Model file for the job. Use its own axes, mm. Face numbers are marked on the shaded views. Give positions to 0.01 mm unless a question says otherwise; leave off trailing zeros. Write each loop counter-clockwise with the first axis right and the second up, starting at its lowest first coordinate (ties: lowest second). Pieces come first, ordered by that corner, then holes. Notation, with made-up numbers: (23.25, 71.25) - (29.25, 71.25) arc R15 cw to (29.25, 80.25) - close; hole circle Ø6 at (11.5, 46). An arc over 180 degrees is marked (long way). Use CSV: the item, a comma, the result in double quotes.
from build123d import *

# Parameters (mm, degrees)
SKETCH1_W               = 245
SKETCH1_H               = 245
BOSS_EXTRUDE1_DEPTH     = 5
SKETCH2_R               = 16.25
CUT_EXTRUDE1_DEPTH      = 10
SKETCH3_R               = 9
CUT_EXTRUDE2_DEPTH      = 10
SKETCH3_3_R             = 9
CUT_EXTRUDE3_DEPTH      = 6
CUT_EXTRUDE3_DEPTH_BACK = 6


with BuildPart() as part:
    # Sketch1 → Boss-Extrude1 (new body, symmetric)
    with BuildSketch(Plane(origin=(0, 0, 0), x_dir=(1, 0, 0), z_dir=(0, 1, 0))):
        Rectangle(SKETCH1_W, SKETCH1_H)
    extrude(amount=BOSS_EXTRUDE1_DEPTH, both=True)

    # Sketch2 → Cut-Extrude1 (cut)
    with BuildSketch(Plane(origin=(0, 5, 0), x_dir=(1, 0, 0), z_dir=(0, 1, 0))):
        with Locations((-66.25, 76.25)):
            Circle(SKETCH2_R)
        with Locations((66.25, 76.25)):
            Circle(SKETCH2_R)
    extrude(amount=-CUT_EXTRUDE1_DEPTH, mode=Mode.SUBTRACT)

    # Sketch3 → Cut-Extrude2 (cut)
    with BuildSketch(Plane(origin=(0, 0, 0), x_dir=(1, 0, 0), z_dir=(0, 1, 0))):
        with Locations((71.5, -103.5)):
            Circle(SKETCH3_R)
    extrude(amount=-CUT_EXTRUDE2_DEPTH, mode=Mode.SUBTRACT)

    # Sketch3<3> → Cut-Extrude3 (cut, two sides)
    with BuildSketch(Plane(origin=(0, 0, 0), x_dir=(1, 0, 0), z_dir=(0, 1, 0))) as cut_extrude3_sk:
        with Locations((103.5, -88.5)):
            Circle(SKETCH3_3_R)
        with Locations((71.5, -103.5)):
            Circle(SKETCH3_3_R)
        with Locations((-71.5, -103.5)):
            Circle(SKETCH3_3_R)
        with Locations((-103.5, -88.5)):
            Circle(SKETCH3_3_R)
    extrude(amount=CUT_EXTRUDE3_DEPTH, mode=Mode.SUBTRACT)
    extrude(cut_extrude3_sk.sketch, amount=-CUT_EXTRUDE3_DEPTH_BACK, mode=Mode.SUBTRACT)


solid = part.part
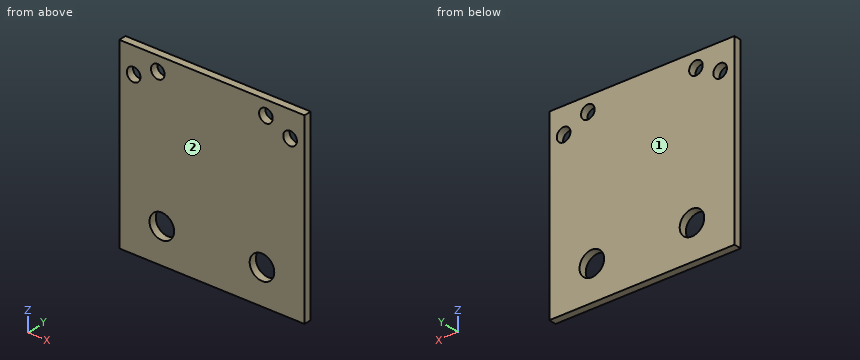
(1) Saw through at A-A, the plane z = 88.5. List the corners of the cut face in (x, y), then the cut area to 3 significant figures.
Checked values:
outline,"(-122.5, -5) - (-112.5, -5) - (-112.5, 5) - (-122.5, 5) - close; (-94.5, -5) - (94.5, -5) - (94.5, 5) - (-94.5, 5) - close; (112.5, -5) - (122.5, -5) - (122.5, 5) - (112.5, 5) - close"
area,"2,090 mm^2"
(2) Saw through at D-D, the plane z = -76.25. List the corners of the cut face in (x, y), then the cut area to 3 significant figures.
Checked values:
outline,"(-122.5, -5) - (-82.5, -5) - (-82.5, 5) - (-122.5, 5) - close; (-50, -5) - (50, -5) - (50, 5) - (-50, 5) - close; (82.5, -5) - (122.5, -5) - (122.5, 5) - (82.5, 5) - close"
area,"1,800 mm^2"
(3) Saw through at C-C, the plane x = -103.5. List the corners of the cut face in (y, z), then the cut area to 3 significant figures.
Checked values:
outline,"(-5, -122.5) - (5, -122.5) - (5, 79.5) - (-5, 79.5) - close; (-5, 97.5) - (5, 97.5) - (5, 122.5) - (-5, 122.5) - close"
area,"2,270 mm^2"
(4) Saw through at B-B, the plane y = 3. List the corners of the cut face in (x, z), then the cut area to 3 significant figures.
Checked values:
outline,"(-122.5, -122.5) - (122.5, -122.5) - (122.5, 122.5) - (-122.5, 122.5) - close; hole circle Ø18 at (-103.5, 88.5); hole circle Ø32.5 at (-66.25, -76.25); hole circle Ø18 at (-71.5, 103.5); hole circle Ø32.5 at (66.25, -76.25); hole circle Ø18 at (71.5, 103.5); hole circle Ø18 at (103.5, 88.5)"
area,"57,300 mm^2"
(5) Pull direction Y, two halves, no side cores. Call the marked faces 1 and 2: released by +Y, released by -Y, zero draft, split by the parting line, or undercut.
Checked values:
face 1,"released by +Y"
face 2,"released by -Y"
(6) Wall check: probe 1 along X at (y, z) = (0, 88.5); probe 2 along Z at (x, y) = (-66.25, -1.25); probe 3 along Z at (x, y) = (71.5, -2.25). Give the ranges that are in metal, low to high. Write a range as [from, to].
Checked values:
probe 1,"x = [-122.5, -112.5], [-94.5, 94.5], [112.5, 122.5]"
probe 2,"z = [-122.5, -92.5], [-60, 96.19], [110.81, 122.5]"
probe 3,"z = [-122.5, -91.63], [-60.87, 94.5], [112.5, 122.5]"
